Solid Edge part; units mm, degrees
sketch "Sketch1" plane through (0, 0, 0) normal (0, 0, 1) x (1, 0, 0)
  line L0 (-30, 35) -> (-30, 0)
  line L1 (-30, 0) -> (30, 0)
  line L2 (30, 0) -> (30, 35)
  line L3 (30, 35) -> (10, 50)
  line L4 (10, 50) -> (-10, 50)
  line L5 (-10, 50) -> (-30, 35)
  dimension "D1" = 30
  dimension "D2" = 30
extrude "Protrusion1" add sketch "Sketch1" along normal mid plane 6
chamfer "Chamfer_1" distance 1 angle 45 6 edges at (-30, 17.5, 3) (0, 0, 3) (-20, 42.5, 3) (0, 50, 3) (20, 42.5, 3) (30, 17.5, 3)
hole "Hole_1" at (10, 40, 3) direction (0, 0, -1) diameter 4 end up to next
hole "Hole1" at (-10, 40, 3) direction (0, 0, -1) diameter 4 end up to next
hole "Hole2" at (20, 5, 3) direction (0, 0, -1) diameter 4 end up to next
hole "Hole3" at (-20, 5, 3) direction (0, 0, -1) diameter 4 end up to next
sketch "Sketch2" plane through (-10, 0, 0) normal (1, 0, 0) x (0, 1, 0)
  line L0 (30.15, 3) -> (20, 3)
  line L1 (30.15, -1.6) -> (30.15, 3)
  line L2 (26.6, -1.6) -> (30.15, -1.6)
  line L3 (26.6, -3) -> (26.6, -1.6)
  line L4 (20, -3) -> (26.6, -3)
  dimension "D1" = 40
  dimension "D2" = 26.6
revolve "RevolvedCutout1" cut sketch "Sketch2" angle 360 about axis through (-10, 20, -3) along (0, 0, 1)
sketch "Sketch3" plane through (0, 25, 3) normal (0, 0, 1) x (1, 0, 0)
  line L0 (-10, -15.15) -> (20.15, -15.15)
  line L1 (20.15, -15.15) -> (20.15, 5.15)
  line L2 (20.15, 5.15) -> (-10, 5.15)
  line L3 (-10, 5.15) -> (-10, -15.15)
  dimension "D1" = 20.15
extrude "Cutout1" cut sketch "Sketch3" against normal up to vertex (4.6 mm away)
sketch "Sketch4" plane through (0, 25, 3) normal (0, 0, 1) x (1, 0, 0)
  line L0 (0.15, -15.15) -> (-20.15, -15.15)
  line L1 (-20.15, -15.15) -> (-20.15, 5.15)
  line L2 (-20.15, 5.15) -> (0.15, 5.15)
  line L3 (0.15, 5.15) -> (0.15, -15.15)
extrude "Cutout2" cut sketch "Sketch4" against normal blind 2.1
hole "Hole_5" at (25.15, 25, 3) direction (0, 0, -1) diameter 4 end up to next
hole "Hole4" at (25.15, 15, 3) direction (0, 0, -1) diameter 4 end up to next
chamfer "Chamfer_2" distance 0.5 angle 45 10 edges at (-10, 42, 3) (10, 42, 3) (25.15, 27, 3) (25.15, 17, 3) (20, 7, 3) (-20, 7, 3) (0, 30.15, 3) (20.15, 20, 3) (0, 9.85, 3) (-20.15, 20, 3)
sketch "Sketch5" plane through (0, 25, 3) normal (0, 0, 1) x (1, 0, 0)
  line L0 (20.15, -4) -> (30, -4)
  line L1 (30, -4) -> (30, -6)
  line L2 (30, -6) -> (20.15, -6)
  line L3 (20.15, -6) -> (20.15, -4)
  dimension "D1" = 30
extrude "ExtrudedCutout_3" cut sketch "Sketch5" against normal blind 3
mirror "Mirror1" about plane through (0, 0, 0) normal (1, 0, 0) of "Hole_5", "Hole4", "ExtrudedCutout_3"
chamfer "Chamfer1" distance 0.5 angle 45 2 edges at (-25.15, 27, 3) (-25.15, 17, 3)
sketch "Sketch6" plane through (0, 25, 3) normal (0, 0, 1) x (1, 0, 0)
  line L0 (-30, -6) -> (-30, -4)
  line L1 (-30, -4) -> (-18, -4)
  line L2 (-18, -4) -> (-18, -6)
  line L3 (-18, -6) -> (-30, -6)
  dimension "D1" = 18
  dimension "D2" = 18
extrude "ExtrudedCutout_5" cut sketch "Sketch6" against normal blind 3
properties material "Polyethylene, low density"
Verification items for the finished model (mm, model axes). A direction names the side the tool comes from. Coordinates: 2 decimals unless noted, no trailing zeros. Order: outer loops, then holes, each group sorted by start corner. A loop starts at its lowest first (then second) coordinate and runs counter-clockwise, first axis right, second up.
Item 1: Section check C-C, the plane x = -25.15. Enter the section's corners in (y, z), then the cut area to 3 significant figures.
Filled in:
outline: (0, -3) - (13, -3) - (13, 2.5) - (12.5, 3) - (1, 3) - (0, 2) - close; (17, -3) - (23, -3) - (23, 2.5) - (22.5, 3) - (21, 3) - (21, 0) - (19, 0) - (19, 3) - (17.5, 3) - (17, 2.5) - close; (27, -3) - (38.64, -3) - (38.64, 2) - (37.39, 3) - (27.5, 3) - (27, 2.5) - close
area: 176 mm2
Item 2: Section check B-B, the plane y = 25. Give the number of separate pieces and of enclosed holes in the cut face, then the cut area to 3 significant figures.
Filled in:
separate pieces: 4
enclosed holes: 0
area: 116 mm2
Item 3: Section check D-D, the plane x = 6.5. Enter the section's corners in (y, z), then the cut area to 3 significant figures.
Filled in:
outline: (0, -3) - (50, -3) - (50, 2) - (49, 3) - (30.65, 3) - (30.15, 2.5) - (30.15, -1.6) - (9.85, -1.6) - (9.85, 2.5) - (9.35, 3) - (1, 3) - (0, 2) - close
area: 205 mm2
Item 4: Access from +Z, -Z, +X, -X, +Y, -Y to the whole of each face (thin tool, end or side, straight path). Record for faces 4 (the face through (20.14, 42.395, -0.535)), 5 (the face through (4, 20, -1.6)), 6 (the face through (-25, 19, 2)).
Filled in:
face 4: +Z, -Z, +X, +Y
face 5: +Z
face 6: +Z, +X, -X
Item 5: Section check A-A, the plane y = 40. Enter the section's corners in (x, z), then the cut area to 3 significant figures.
Filled in:
outline: (-23.33, -3) - (-12, -3) - (-12, 2.5) - (-12.5, 3) - (-21.67, 3) - (-23.33, 2) - close; (-8, -3) - (8, -3) - (8, 2.5) - (7.5, 3) - (-7.5, 3) - (-8, 2.5) - close; (12, -3) - (23.33, -3) - (23.33, 2) - (21.67, 3) - (12.5, 3) - (12, 2.5) - close
area: 230 mm2
Item 6: Material ranges on L1, parallel to Y at x = 10, z = 0.9; L2, parallel to X at y = 15, z = 1.45; L3, parallel to X at y = 5, z = -1.8, recorded low to high.
Filled in:
L1: y = 0 to 9.85, 30.15 to 38, 42 to 50
L2: x = -30 to -27.15, -23.15 to -20.15, 20.15 to 23.15, 27.15 to 30
L3: x = -30 to -22, -18 to 18, 22 to 30
Item 7: Release check for a two-part mould opening along X. For faces 1 (the face through (0, 0, -1)), 2 (the face through (-18, 12, 0.9)), 3 (the face through (19.844, 42.001, 2.493)) record: +X half, -X half, draft (parallel to the pull), parting line (faces both ways), or undercut.
Filled in:
face 1: draft
face 2: undercut
face 3: +X half
Item 8: Depth check by flat-ended pin: pin 1 (15 mm diameter, centred on x = -10, y = 20, fed in from +Z); pin 2 (3.5 mm diameter, centred on x = 27, z = 1, fed in from +Y); pin 3 (1.5 mm diameter, centred on x = -27.5, z = 1.5, fed in from +Y). Enter the tip coordinate at first touch or a pass-through.
Filled in:
pin 1: stops at z = -1.6
pin 2: stops at y = 38.56
pin 3: stops at y = 37.44
